Check sheet for the modelled part. Datum: model origin and axes. Units: mm. Give positions to 0.01 mm unless a question says otherwise; leave off trailing zeros. Loops run counter-clockwise (first coordinate to the right, second up) from the corner with the lowest first, then second, coordinate; pieces in that order, holes last.
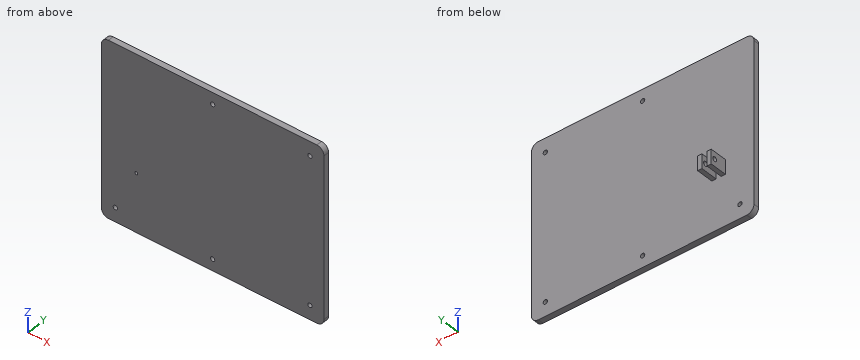
```python
from build123d import *

# Parameters (mm, degrees)
SKETCH1_W           = 248.69467868
SKETCH1_H           = 191.562117362
BOSS_EXTRUDE1_DEPTH = 4
CUT_EXTRUDE1_DEPTH  = 10
SKETCH3_R           = 1.5
CUT_EXTRUDE2_DEPTH  = 4
SKETCH10_W          = 3
SKETCH10_H          = 10
BOSS_EXTRUDE2_DEPTH = 12
SKETCH12_R          = 1.6
CUT_EXTRUDE3_DEPTH  = 10
SKETCH13_R          = 1
CUT_EXTRUDE4_DEPTH  = 6


with BuildPart() as part:
    # Sketch1 → Boss-Extrude1 (new body)
    with BuildSketch(Plane(origin=(0, 0, 0), x_dir=(1, 0, 0), z_dir=(0, 1, 0))):
        Rectangle(SKETCH1_W, SKETCH1_H)
    extrude(amount=BOSS_EXTRUDE1_DEPTH)

    # Sketch2 → Cut-Extrude1 (cut)
    with BuildSketch(Plane(origin=(0, 4, 0), x_dir=(1, 0, 0), z_dir=(0, 1, 0))):
        with BuildLine():
            Line((-53.628035699, 20.218941319), (-53.628035699, -90.781058681))
            ThreePointArc((-53.628035699, -90.781058681), (-52.163569604, -94.316592587), (-48.628035699, -95.781058681))
            Line((-48.628035699, -95.781058681), (-124.34733934, -95.781058681))
            Line((-124.34733934, -95.781058681), (-124.34733934, 95.781058681))
            Line((-124.34733934, 95.781058681), (124.34733934, 95.781058681))
            Line((124.34733934, 95.781058681), (124.34733934, -95.781058681))
            Line((124.34733934, -95.781058681), (97.371964301, -95.781058681))
            ThreePointArc((97.371964301, -95.781058681), (100.907498207, -94.316592587), (102.371964301, -90.781058681))
            Line((102.371964301, -90.781058681), (102.371964301, 20.218941319))
            ThreePointArc((102.371964301, 20.218941319), (100.907498207, 23.754475225), (97.371964301, 25.218941319))
            Line((97.371964301, 25.218941319), (-48.628035699, 25.218941319))
            ThreePointArc((-48.628035699, 25.218941319), (-52.163569604, 23.754475225), (-53.628035699, 20.218941319))
        make_face()
    extrude(amount=-CUT_EXTRUDE1_DEPTH, mode=Mode.SUBTRACT)

    # Sketch3 → Cut-Extrude2 (cut)
    with BuildSketch(Plane(origin=(0, 4, 0), x_dir=(1, 0, 0), z_dir=(0, 1, 0))):
        with Locations((-43.82473484, 15.41564046)):
            Circle(SKETCH3_R)
        with Locations((24.371964301, 17.218941319)):
            Circle(SKETCH3_R)
        with Locations((92.568663443, 15.41564046)):
            Circle(SKETCH3_R)
        with Locations((24.371964301, -87.781058681)):
            Circle(SKETCH3_R)
        with Locations((92.568663443, -85.977757822)):
            Circle(SKETCH3_R)
    extrude(amount=-CUT_EXTRUDE2_DEPTH, mode=Mode.SUBTRACT)

    # Sketch10 → Boss-Extrude2 (add)
    with BuildSketch(Plane(origin=(0, 4, 0), x_dir=(1, 0, 0), z_dir=(0, 1, 0))):
        with Locations((-32.128035699, -14.781058681)):
            Rectangle(SKETCH10_W, SKETCH10_H)
        with Locations((-25.628035699, -14.781058681)):
            Rectangle(SKETCH10_W, SKETCH10_H)
    extrude(amount=BOSS_EXTRUDE2_DEPTH)

    # Sketch12 → Cut-Extrude3 (cut)
    with BuildSketch(Plane.ZY.offset(33.628035699)):
        with Locations((14.781058681, 13)):
            Circle(SKETCH12_R)
    extrude(amount=-CUT_EXTRUDE3_DEPTH, mode=Mode.SUBTRACT)

    # Sketch13 → Cut-Extrude4 (cut)
    with BuildSketch(Plane(origin=(0, 4, 0), x_dir=(1, 0, 0), z_dir=(0, 1, 0))):
        with Locations((-29.127206005, -15.029218682)):
            Circle(SKETCH13_R)
    extrude(amount=-CUT_EXTRUDE4_DEPTH, mode=Mode.SUBTRACT)


solid = part.part
```
(1) Material ranges on line 1 (Y direction, x = -44, z = 17.5), recorded low to high.
(2) Section check B-B on x = -0.5. Record the boundary of the cut face in (y, z), plus the area to 3 significant figures.
(3) Gauge pin test, flat ends, axial feed: pin 1 Ø2.5 at (x, y) = (-32, 7.5) entering from -Z; pin 2 Ø3 at (y, z) = (11, 14) entering from -X; pin 3 Ø1.5 at (x, y) = (-25, 10) entering from +Z. Record the tip position at first contact, or that the pin passes through.
(4) Section check C-C on z = 81. Record the boundary of the cut face in (x, y).
(5) Section check A-A on y = 8. Record the boundary of the cut face in (x, z).
Computed values:
1. line 1: y = 0 to 4
2. outline: (0, -25.22) - (4, -25.22) - (4, 95.78) - (0, 95.78) - close
2. area: 484 mm2
3. pin 1: stops at z = 9.78
3. pin 2: stops at x = -33.63
3. pin 3: stops at z = 19.78
4. outline: (-53.63, 0) - (102.37, 0) - (102.37, 4) - (-53.63, 4) - close
5. outline: (-33.63, 9.78) - (-30.63, 9.78) - (-30.63, 19.78) - (-33.63, 19.78) - close; (-27.13, 9.78) - (-24.13, 9.78) - (-24.13, 19.78) - (-27.13, 19.78) - close
